The listing builds one solid part. Answer for the finished solid, in the listing's coordinates (mm). A direction names the side the tool comes from. Give positions to 0.01 mm unless a question says otherwise; leave off trailing zeros. Write each loop counter-clockwise with the first axis right and the second up, starting at its lowest first coordinate (ties: lowest second). Pieces come first, ordered by that corner, then holes. Notation, with made-up numbers: (49, 20.5) - (107, 20.5) arc R37 cw to (107, 58.5) - close; hole circle Ø1 at (47, 64.25). An arc over 180 degrees is marked (long way). Answer as CSV lines item,"result". Start each with the question number.
(1) For a pull along X with two mould halves and no side action, classify faces 1 (the face through (17.4, -17.43, 15.44)), 2 (the face through (14.93, 14.9, 15.32)), 3 (the face through (0, 18, 15)) as pulls with the +X half, pulls with the -X half, needs draft (parallel to the pull), parting line crosses it, or undercut.
(2) Find section A-A (z = 15.5). Write down the section's boundary in (x, y).
(3) For faces 4 (the face through (-17.43, 17.4, 15.44)), 5 (the face through (18, 0, 15)), 6 (the face through (-0.189, 15.864, 29.479)), determine the directions among +Z, -Z, +X, -X, +Y, -Y from which every point of the face is accessible in a straight line to the end or side of a thin tool.
(4) Find section B-B (y = -7). Write down the section's boundary in (x, z).
(5) Straight lines are drawn through the part: probe 1 along Y at (x, z) = (-4.5, 19); probe 2 along Z at (x, y) = (13, 0). For each, find the intervals that lie inside material, in ascending order.
(6) Each of these flat-tipped pins is pushed along its axis until it touches: pin 1 Ø10 at (y, z) = (8, 12) entering from -X; pin 2 Ø4 at (x, y) = (5, 8) entering from +Z; pin 3 Ø8 at (x, y) = (13.5, 8) entering from +Z. Where does it stop, or does it pass through?
from build123d import *

# Parameters (mm, degrees)
F0_W         = 36
F0_H         = 36
F1_DEPTH     = 2
F2_DEPTH     = 30
F3_T         = -2.5
F4_R         = 2
F5_T1_DEPTH  = 32
F5_T3_DEPTH  = 27
F5_T5_DEPTH  = 32
F5_T7_DEPTH  = 27
F5_T10_ANGLE = 90
F5_T12_ANGLE = 90
F5_T14_ANGLE = 90
F5_T16_ANGLE = 90
F5_T18_ANGLE = 90
F5_T20_ANGLE = 90
F5_T22_ANGLE = 90
F5_T24_ANGLE = 90


# Not quite as in the source:
# - a fillet or chamfer that OpenCascade refuses, or shapes differently, is made with other operations: its cross-section is extruded or revolved along the edge and cut away or added


with BuildPart() as f1:
    # F0 (on Top) → F1 (new body)
    with BuildSketch(Plane.XY):
        with BuildLine():
            ThreePointArc((20, 18), (19.4142135624, 19.4142135624), (18, 20))
            Line((18, 20), (-18, 20))
            ThreePointArc((-18, 20), (-19.4142135624, 19.4142135624), (-20, 18))
            Line((-20, 18), (-20, -18))
            ThreePointArc((-20, -18), (-19.4142135624, -19.4142135624), (-18, -20))
            Line((-18, -20), (18, -20))
            ThreePointArc((18, -20), (19.4142135624, -19.4142135624), (20, -18))
            Line((20, -18), (20, 18))
        make_face()
        Rectangle(F0_W, F0_H, mode=Mode.SUBTRACT)
    extrude(amount=F1_DEPTH)

    # F0 (on Top) → F2 (join)
    with BuildSketch(Plane.XY):
        Rectangle(F0_W, F0_H)
    extrude(amount=F2_DEPTH)

    # F3
    f3_openings = [f1.faces().sort_by_distance(p)[0] for p in [
        (0, 0, 30),
    ]]
    offset(amount=F3_T, openings=f3_openings)

    # F4
    f4_edges = [f1.edges().sort_by_distance(p)[0] for p in [
        (-18, -18, 16),
        (18, 18, 16),
        (-18, 18, 16),
        (18, -18, 16),
        (-15.5, -15.5, 16.25),
        (15.5, -15.5, 16.25),
        (15.5, 15.5, 16.25),
        (-15.5, 15.5, 16.25),
    ]]
    fillet(f4_edges, radius=F4_R)

    # F5: fillet of radius 1.5 on 16 edges, made by hand

    # F5_s2 → F5_t1 (cut)
    with BuildSketch(Plane.XZ.offset(-16)):
        with BuildLine():
            ThreePointArc((-18, 28.5), (-17.5606601718, 29.5606601718), (-16.5, 30))
            Line((-16.5, 30), (-18, 30))
            Line((-18, 30), (-18, 28.5))
        make_face()
        with BuildLine():
            ThreePointArc((18, 28.5), (17.5606601718, 29.5606601718), (16.5, 30))
            Line((16.5, 30), (18, 30))
            Line((18, 30), (18, 28.5))
        make_face()
    extrude(amount=F5_T1_DEPTH, mode=Mode.SUBTRACT)

    # F5_s4 → F5_t3 (cut)
    with BuildSketch(Plane.XZ.offset(-13.5)):
        with BuildLine():
            ThreePointArc((-17, 30), (-15.9393398282, 29.5606601718), (-15.5, 28.5))
            Line((-15.5, 28.5), (-15.5, 30))
            Line((-15.5, 30), (-17, 30))
        make_face()
        with BuildLine():
            ThreePointArc((17, 30), (15.9393398282, 29.5606601718), (15.5, 28.5))
            Line((15.5, 28.5), (15.5, 30))
            Line((15.5, 30), (17, 30))
        make_face()
    extrude(amount=F5_T3_DEPTH, mode=Mode.SUBTRACT)

    # F5_s6 → F5_t5 (cut)
    with BuildSketch(Plane.YZ.offset(-16)):
        with BuildLine():
            ThreePointArc((18, 28.5), (17.5606601718, 29.5606601718), (16.5, 30))
            Line((16.5, 30), (18, 30))
            Line((18, 30), (18, 28.5))
        make_face()
        with BuildLine():
            ThreePointArc((-18, 28.5), (-17.5606601718, 29.5606601718), (-16.5, 30))
            Line((-16.5, 30), (-18, 30))
            Line((-18, 30), (-18, 28.5))
        make_face()
    extrude(amount=F5_T5_DEPTH, mode=Mode.SUBTRACT)

    # F5_s8 → F5_t7 (cut)
    with BuildSketch(Plane.YZ.offset(-13.5)):
        with BuildLine():
            ThreePointArc((-17, 30), (-15.9393398282, 29.5606601718), (-15.5, 28.5))
            Line((-15.5, 28.5), (-15.5, 30))
            Line((-15.5, 30), (-17, 30))
        make_face()
        with BuildLine():
            ThreePointArc((17, 30), (15.9393398282, 29.5606601718), (15.5, 28.5))
            Line((15.5, 28.5), (15.5, 30))
            Line((15.5, 30), (17, 30))
        make_face()
    extrude(amount=F5_T7_DEPTH, mode=Mode.SUBTRACT)

    # F5_s9 → F5_t10 (revolve, cut)
    with BuildSketch(Plane.YZ.offset(-16)):
        with BuildLine():
            ThreePointArc((18, 28.5), (17.5606601718, 29.5606601718), (16.5, 30))
            Line((16.5, 30), (18, 30))
            Line((18, 30), (18, 28.5))
        make_face()
    revolve(axis=Axis((-16, 16, 30), (0, 0, 1)), revolution_arc=F5_T10_ANGLE, mode=Mode.SUBTRACT)

    # F5_s11 → F5_t12 (revolve, cut)
    with BuildSketch(Plane.YZ.offset(16)):
        with BuildLine():
            ThreePointArc((18, 28.5), (17.5606601718, 29.5606601718), (16.5, 30))
            Line((16.5, 30), (18, 30))
            Line((18, 30), (18, 28.5))
        make_face()
    revolve(axis=Axis((16, 16, 30), (0, 0, -1)), revolution_arc=F5_T12_ANGLE, mode=Mode.SUBTRACT)

    # F5_s13 → F5_t14 (revolve, cut)
    with BuildSketch(Plane.YZ.offset(-16)):
        with BuildLine():
            ThreePointArc((-18, 28.5), (-17.5606601718, 29.5606601718), (-16.5, 30))
            Line((-16.5, 30), (-18, 30))
            Line((-18, 30), (-18, 28.5))
        make_face()
    revolve(axis=Axis((-16, -16, 30), (0, 0, -1)), revolution_arc=F5_T14_ANGLE, mode=Mode.SUBTRACT)

    # F5_s15 → F5_t16 (revolve, cut)
    with BuildSketch(Plane.XZ.offset(16)):
        with BuildLine():
            ThreePointArc((18, 28.5), (17.5606601718, 29.5606601718), (16.5, 30))
            Line((16.5, 30), (18, 30))
            Line((18, 30), (18, 28.5))
        make_face()
    revolve(axis=Axis((16, -16, 30), (0, 0, -1)), revolution_arc=F5_T16_ANGLE, mode=Mode.SUBTRACT)

    # F5_s17 → F5_t18 (revolve, cut)
    with BuildSketch(Plane.XZ.offset(13.5)):
        with BuildLine():
            ThreePointArc((17, 30), (15.9393398282, 29.5606601718), (15.5, 28.5))
            Line((15.5, 28.5), (15.5, 30))
            Line((15.5, 30), (17, 30))
        make_face()
    revolve(axis=Axis((13.5, -13.5, 30), (0, 0, -1)), revolution_arc=F5_T18_ANGLE, mode=Mode.SUBTRACT)

    # F5_s19 → F5_t20 (revolve, cut)
    with BuildSketch(Plane.XZ.offset(-13.5)):
        with BuildLine():
            ThreePointArc((17, 30), (15.9393398282, 29.5606601718), (15.5, 28.5))
            Line((15.5, 28.5), (15.5, 30))
            Line((15.5, 30), (17, 30))
        make_face()
    revolve(axis=Axis((13.5, 13.5, 30), (0, 0, 1)), revolution_arc=F5_T20_ANGLE, mode=Mode.SUBTRACT)

    # F5_s21 → F5_t22 (revolve, cut)
    with BuildSketch(Plane.XZ.offset(13.5)):
        with BuildLine():
            ThreePointArc((-17, 30), (-15.9393398282, 29.5606601718), (-15.5, 28.5))
            Line((-15.5, 28.5), (-15.5, 30))
            Line((-15.5, 30), (-17, 30))
        make_face()
    revolve(axis=Axis((-13.5, -13.5, 30), (0, 0, 1)), revolution_arc=F5_T22_ANGLE, mode=Mode.SUBTRACT)

    # F5_s23 → F5_t24 (revolve, cut)
    with BuildSketch(Plane.YZ.offset(-13.5)):
        with BuildLine():
            ThreePointArc((17, 30), (15.9393398282, 29.5606601718), (15.5, 28.5))
            Line((15.5, 28.5), (15.5, 30))
            Line((15.5, 30), (17, 30))
        make_face()
    revolve(axis=Axis((-13.5, 13.5, 30), (0, 0, 1)), revolution_arc=F5_T24_ANGLE, mode=Mode.SUBTRACT)


solid = f1.part
Result set:
1,face 1,"pulls with the +X half"
1,face 2,"undercut"
1,face 3,"needs draft"
2,outline,"(-18, -16) arc R2 ccw to (-16, -18) - (16, -18) arc R2 ccw to (18, -16) - (18, 16) arc R2 ccw to (16, 18) - (-16, 18) arc R2 ccw to (-18, 16) - close; hole (-15.5, -13.5) arc R2 ccw to (-13.5, -15.5) - (13.5, -15.5) arc R2 ccw to (15.5, -13.5) - (15.5, 13.5) arc R2 ccw to (13.5, 15.5) - (-13.5, 15.5) arc R2 ccw to (-15.5, 13.5) - close"
3,face 4,"+Z, -X, +Y"
3,face 5,"+Z, +X, +Y, -Y"
3,face 6,"+Z"
4,outline,"(-20, 0) - (20, 0) - (20, 2) - (18, 2) - (18, 28.5) arc R1.5 ccw to (16.75, 29.98) arc R1.5 ccw to (15.5, 28.5) - (15.5, 2.5) - (-15.5, 2.5) - (-15.5, 28.5) arc R1.5 ccw to (-16.75, 29.98) arc R1.5 ccw to (-18, 28.5) - (-18, 2) - (-20, 2) - close"
5,probe 1,"-18 to -15.5, 15.5 to 18"
5,probe 2,"0 to 2.5"
6,pin 1,"x = -18"
6,pin 2,"z = 2.5"
6,pin 3,"z = 29.98"
